Build history of the part. All positions in model axes, mm. Face numbers are marked on the shaded views. Round coordinates to 2 decimals unless told otherwise and drop trailing zeros. Write each loop counter-clockwise with the first axis right and the second up, starting at its lowest first coordinate (ties: lowest second). Pieces come first, ordered by that corner, then holes. Notation, with made-up numbers: (27, 4.5) -> (42, 4.5) arc R9 cw to (42, 8.5) -> close; hole circle Ø1 at (-6, 47.25). An arc over 180 degrees is marked (long way). Answer in a Markdown table with one row per item.
Autodesk Inventor part; units mm, degrees
ref_plane "YZ Plane" through (0, 0, 0) normal (1, 0, 0) x (0, 1, 0)
ref_plane "XZ Plane" through (0, 0, 0) normal (0, 1, 0) x (-1, 0, 0)
ref_plane "XY Plane" through (0, 0, 0) normal (0, 0, 1) x (1, 0, 0)
sketch "Sketch1" plane through (0, 0, 0) normal (1, 0, 0) x (0, 1, 0)
  line L0 (60.5, 1.15) -> (-60.5, 1.15)
  line L1 (-60.5, 1.15) -> (-60.5, -1.15)
  line L2 (-60.5, -1.15) -> (60.5, -1.15)
  line L3 (60.5, -1.15) -> (60.5, 1.15)
  line L4 (60.5, 1.15) -> (-60.5, -1.15) construction
  line L5 (-60.5, 1.15) -> (60.5, -1.15) construction
  line L6 (60.5, -1.15) -> (81.7132, 20.0632)
  line L7 (60.5, -1.15) -> (90.5, -1.15) construction
  line L8 (81.7132, 20.0632) -> (80.0869, 21.6895)
  line L9 (80.0869, 21.6895) -> (59.5288, 1.1315)
  line L10 (80.0869, 21.6895) -> (100.0869, 21.6895)
  line L11 (100.0869, 21.6895) -> (100.0869, 19.3895)
  line L12 (100.0869, 19.3895) -> (81.0395, 19.3895)
  line L13 (100.0869, 19.3895) -> (102.3869, 19.3895)
  line L14 (102.3869, 19.3895) -> (102.3869, 120.8895)
  line L15 (102.3869, 120.8895) -> (100.0869, 120.8895)
  line L16 (100.0869, 120.8895) -> (100.0869, 19.3895)
  line L17 (102.3869, 120.8895) -> (82.3869, 120.8895)
  line L18 (82.3869, 120.8895) -> (82.3869, 116.8895)
  line L19 (82.3869, 116.8895) -> (102.3869, 116.8895)
  line L20 (102.3869, 116.8895) -> (102.3869, 120.8895)
  point P0 (0, 0)
  point P1 (59.5473, 1.15)
  point P2 (100.0869, 116.8895)
  point P3 (100.0869, 21.6895)
  dimension "d0" = 121
  dimension "d1" = 2.3
  dimension "d2" = 30
  dimension "d3" = 45
  dimension "d4" = 2.3
  dimension "d5" = 20
  dimension "d6" = 2.3
  dimension "d7" = 2.3
  dimension "d8" = 101.5
  dimension "d9" = 20
  dimension "d10" = 4
extrude "Extrusion1" add sketch "Sketch1" against normal blind 239
fillet "Fillet1" radius 4 1 edges at (-119.5, 60.5, -1.15)
fillet "Fillet2" radius 4 5 edges at (-119.5, 59.5473, 1.15) (-119.5, 81.0395, 19.3895) (-119.5, 80.0869, 21.6895) (-119.5, 102.3869, 120.8895) (-119.5, 100.0869, 116.8895)
sketch "Sketch2" plane through (0, -60.5, -1.15) normal (0, 0, -1) x (-1, 0, 0)
  line L0 (22, -20) -> (217, -20)
  line L1 (217, -20) -> (217, 20)
  line L2 (217, 20) -> (22, 20)
  line L3 (22, 20) -> (22, -20)
  line L4 (0, 0) -> (239, 0)
  line L5 (22, -20) -> (217, 20) construction
  line L6 (217, -20) -> (22, 20) construction
  line L7 (239, 119.3431) -> (239, 0)
  line L8 (0, 0) -> (0, 119.3431)
  line L9 (119.5, 20) -> (119.5, 119.3431) construction
  line L10 (119.5, 119.3431) -> (119.5, 0) construction
  line L11 (32, 20) -> (47, 20) construction
  line L12 (47, 20) -> (47, 30)
  line L13 (47, 30) -> (32, 30)
  line L14 (32, 30) -> (32, 20)
  line L15 (32, 20) -> (47, 20) construction
  line L16 (55.3012, 20) -> (70.3012, 20)
  line L17 (94.5, 20) -> (109.5, 20)
  line L18 (109.5, 20) -> (109.5, 30)
  line L19 (109.5, 30) -> (94.5, 30)
  line L20 (94.5, 30) -> (94.5, 20)
  line L21 (63.25, 20) -> (78.25, 20)
  line L22 (78.25, 20) -> (78.25, 30)
  line L23 (78.25, 30) -> (63.25, 30)
  line L24 (63.25, 30) -> (63.25, 20)
  line L25 (47, 30) -> (63.25, 30) construction
  line L26 (78.25, 30) -> (94.5, 30) construction
  line L27 (192, 20) -> (192, 30)
  line L28 (192, 30) -> (207, 30)
  line L29 (207, 30) -> (207, 20)
  line L30 (129.5, 20) -> (129.5, 30)
  line L31 (129.5, 30) -> (144.5, 30)
  line L32 (144.5, 30) -> (144.5, 20)
  line L33 (160.75, 20) -> (160.75, 30)
  line L34 (160.75, 30) -> (175.75, 30)
  line L35 (175.75, 30) -> (175.75, 20)
  point P0 (0, 60.5)
  point P1 (22, 0)
  point P2 (217, 0)
  point P3 (109.5, 20)
  point P4 (192, 20)
  point P5 (207, 20)
  point P6 (160.75, 20)
  dimension "d15" = 195
  dimension "d16" = 40
  dimension "d19" = 22
  dimension "d20" = 22
  dimension "d21" = 15
  dimension "d22" = 10
  dimension "d25" = 15
  dimension "d26" = 10
  dimension "d27" = 10
  dimension "d28" = 10
  dimension "d31" = 15
  dimension "d32" = 10
extrude "Extrusion2" cut sketch "Sketch2" against normal blind 10 contours L3 L2 L1 L4 | L14 L13 L12 L2 | L2 L27 L28 L29 | L2 L33 L34 L35 | L24 L23 L22 L2 | L2 L30 L31 L32 | L20 L19 L18 L2
properties part number "controlbox_cover"
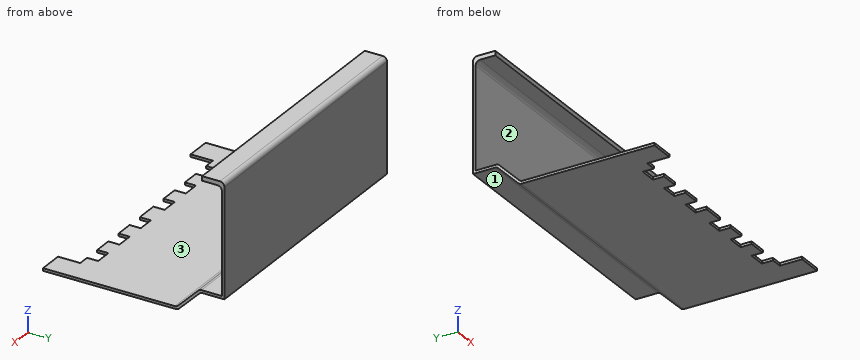
Q1. Saw through at C-C on z = 41.5. Write the cut outline in (x, y).
A:
| item | result |
|---|---|
| outline | (-239, 100.09) -> (0, 100.09) -> (0, 102.39) -> (-239, 102.39) -> close |
Q2. Saw through at D-D on x = -81.5. Write the cut outline in (y, z).
A:
| item | result |
|---|---|
| outline | (-40.5, -1.15) -> (58.84, -1.15) arc R4 ccw to (61.67, 0.02) -> (79.87, 18.22) arc R4 cw to (82.7, 19.39) -> (102.39, 19.39) -> (102.39, 116.89) arc R4 ccw to (98.39, 120.89) -> (82.39, 120.89) -> (82.39, 116.89) -> (96.09, 116.89) arc R4 cw to (100.09, 112.89) -> (100.09, 21.69) -> (81.74, 21.69) arc R4 ccw to (78.92, 20.52) -> (60.72, 2.32) arc R4 cw to (57.89, 1.15) -> (-40.5, 1.15) -> close |
Q3. Drop flat-ended pins along their axis: P1, Ø1.2, axis at x = -213, z = 0, coming from the -Y side; P2, Ø1.8, axis at x = -202.5, z = 0, coming from the -Y side; P3, Ø1.2, axis at x = -72, z = 118, coming from the -Y side. Give the stop position or say it passes through.
A:
| item | result |
|---|---|
| P1 | y = -40.5 |
| P2 | y = -30.5 |
| P3 | y = 82.39 |
Q4. Saw through at B-B on x = -41.5. Write the cut outline in (y, z), plus the area to 3 significant figures.
A:
| item | result |
|---|---|
| outline | (-30.5, -1.15) -> (58.84, -1.15) arc R4 ccw to (61.67, 0.02) -> (79.87, 18.22) arc R4 cw to (82.7, 19.39) -> (102.39, 19.39) -> (102.39, 116.89) arc R4 ccw to (98.39, 120.89) -> (82.39, 120.89) -> (82.39, 116.89) -> (96.09, 116.89) arc R4 cw to (100.09, 112.89) -> (100.09, 21.69) -> (81.74, 21.69) arc R4 ccw to (78.92, 20.52) -> (60.72, 2.32) arc R4 cw to (57.89, 1.15) -> (-30.5, 1.15) -> close |
| area | 624 mm² |
Q5. Wall check: line 1 (Z direction, x = -113, y = 83); line 2 (Y direction, x = -215, z = 25.5); line 3 (Z direction, x = -140.5, y = 40.5). Give the ranges that are in metal, low to high. Write a range as [from, to].
A:
| item | result |
|---|---|
| line 1 | [19.39, 21.69], [116.89, 120.89] |
| line 2 | [100.09, 102.39] |
| line 3 | [-1.15, 1.15] |
Q6. Two-plate mould, pull along Z, no slides. Class the marked faces 1, 2 and 3: released by +Z, released by -Z, zero draft, split by the parting line, or undercut.
A:
| item | result |
|---|---|
| face 1 | released by -Z |
| face 2 | undercut |
| face 3 | released by +Z |
Q7. Saw through at A-A on y = -33.5. Write the cut outline in (x, z).
A:
| item | result |
|---|---|
| outline | (-239, -1.15) -> (-207, -1.15) -> (-207, 1.15) -> (-239, 1.15) -> close; (-192, -1.15) -> (-175.75, -1.15) -> (-175.75, 1.15) -> (-192, 1.15) -> close; (-160.75, -1.15) -> (-144.5, -1.15) -> (-144.5, 1.15) -> (-160.75, 1.15) -> close; (-129.5, -1.15) -> (-109.5, -1.15) -> (-109.5, 1.15) -> (-129.5, 1.15) -> close; (-94.5, -1.15) -> (-78.25, -1.15) -> (-78.25, 1.15) -> (-94.5, 1.15) -> close; (-63.25, -1.15) -> (-47, -1.15) -> (-47, 1.15) -> (-63.25, 1.15) -> close; (-32, -1.15) -> (0, -1.15) -> (0, 1.15) -> (-32, 1.15) -> close |
